For this review, take the finished solid that the model builds, in its own axes (mm). Face numbers are marked on the shaded views. A direction names the side the tool comes from. Round coordinates to 2 decimals unless told otherwise and drop trailing zeros. Write each loop counter-clockwise with the first axis right and the second up, starting at its lowest first coordinate (ties: lowest second). Pieces come first, ordered by that corner, then holes. Notation, with made-up numbers: M 9,81.5 L 24,81.5 A20 cw 24,114.5 Z; hole C 63.25,22 d5. An arc over 180 degrees is marked long. Answer in a Markdown table with one row per item.
Autodesk Fusion 360 part; units mm, degrees
sketch "Sketch1" plane through (0, 0, 0) normal (0, 0, 1) x (1, 0, 0)
  circle A0 centre (0, 0) radius 30
  line L0 (0, 0) -> (129, 0) construction
  circle A1 centre (129, 0) radius 20
  line L1 (-11.547, 20) -> (-23.094, 0)
  line L2 (-23.094, 0) -> (-11.547, -20)
  line L3 (-11.547, -20) -> (11.547, -20)
  line L4 (11.547, -20) -> (23.094, 0)
  line L5 (23.094, 0) -> (11.547, 20)
  line L6 (11.547, 20) -> (-11.547, 20)
  line L7 (0, 0) -> (0, 40) construction
  line L8 (129, 0) -> (129, 50) construction
  line L9 (129, 15) -> (114.7342, 4.6353)
  line L10 (114.7342, 4.6353) -> (120.1832, -12.1353)
  line L11 (120.1832, -12.1353) -> (137.8168, -12.1353)
  line L12 (137.8168, -12.1353) -> (143.2658, 4.6353)
  line L13 (143.2658, 4.6353) -> (129, 15)
  line L14 (28.2843, 10) -> (111.6795, 10)
  line L15 (28.2843, -10) -> (111.6795, -10)
  line L16 (30, 0) -> (109, 0) construction
  line L17 (69.5, 0) -> (69.5, 17.0528) construction
  line L18 (99.5, -5) -> (39.5, -5)
  line L19 (39.5, -5) -> (39.5, 5) construction
  line L20 (39.5, 5) -> (99.5, 5)
  line L21 (99.5, 5) -> (99.5, -5) construction
  line L22 (99.5, -5) -> (39.5, 5) construction
  line L23 (39.5, -5) -> (99.5, 5) construction
  arc A2 (39.5, 5) -> (39.5, -5) centre (39.5, 0) ccw
  arc A3 (99.5, -5) -> (99.5, 5) centre (99.5, 0) ccw
  point P0 (129, 0)
  point P1 (64.5, 0)
  point P2 (69.5, 0)
  dimension "d1" = 60
  dimension "d2" = 129
  dimension "d3" = 40
  dimension "d4" = 20
  dimension "d5" = 15
  dimension "d6" = 10
  dimension "d7" = 10
  dimension "d17" = 10
  dimension "d19" = 60
extrude "Extrude1" add sketch "Sketch1" along normal mid plane 20 contours A0 | A1 makes body 1 at (27.1662, -12.7278, 3.3333) makes body 2 at (148.9006, -1.9914, -3.3333)
extrude "Extrude2" add sketch "Sketch1" along normal mid plane 10 contours A0 A1 L14 L15 bodies 1 2
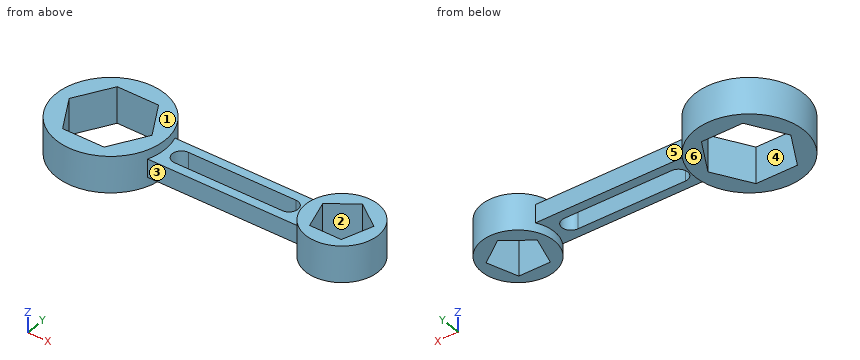
Q1. Take a section at D-D (x = 44). State the section outline as (y, z) points, then the cut area to 3 significant figures.
Found:
| item | result |
|---|---|
| outline | M -10,-5 L -5,-5 L -5,5 L -10,5 Z; M 5,-5 L 10,-5 L 10,5 L 5,5 Z |
| area | 100 mm² |
Q2. Mouldability with a two-part tool opening along X and no side actions: class the marked faces 1 and 2 as +X half, -X half, draft (parallel to the pull), parting line (faces both ways), or undercut.
Found:
| item | result |
|---|---|
| face 1 | draft |
| face 2 | undercut |
Q3. Take a section at B-B (x = 0). State the section outline as (y, z) points, then the cut area to 3 significant figures.
Found:
| item | result |
|---|---|
| outline | M -30,-10 L -20,-10 L -20,10 L -30,10 Z; M 20,-10 L 30,-10 L 30,10 L 20,10 Z |
| area | 400 mm² |
Q4. Machinability: for the marked faces 3, 4, 5 and 6, which of the approach directions +Z, -Z, +X, -X, +Y, -Y give a long, thin tool a straight path to every point of the face, cutting with its end or side? Answer none if there is none.
Found:
| item | result |
|---|---|
| face 3 | +Z, -Z, -Y |
| face 4 | +Z, -Z |
| face 5 | +Z, -Z, +Y |
| face 6 | -Z, +X, -X, +Y, -Y |
Q5. Take a section at A-A (z = -8.25). State the section outline as (x, y) points.
Found:
| item | result |
|---|---|
| outline | C 0,0 d60; C 129,0 d40; hole M -23.09,0 L -11.55,-20 L 11.55,-20 L 23.09,0 L 11.55,20 L -11.55,20 Z; hole M 114.73,4.64 L 120.18,-12.14 L 137.82,-12.14 L 143.27,4.64 L 129,15 Z |
Q6. Take a section at C-C (z = 3). State the section outline as (x, y) points, then the cut area to 3 significant figures.
Found:
| item | result |
|---|---|
| outline | M 28.28,-10 L 111.68,-10 A20 ccw long 111.68,10 L 28.28,10 A30 ccw long Z; hole M -23.09,0 L -11.55,-20 L 11.55,-20 L 23.09,0 L 11.55,20 L -11.55,20 Z; hole M 39.5,-5 L 99.5,-5 A5 ccw 99.5,5 L 39.5,5 A5 ccw Z; hole M 114.73,4.64 L 120.18,-12.14 L 137.82,-12.14 L 143.27,4.64 L 129,15 Z |
| area | 3,090 mm² |
Q7. For probe 1 along X at (y, z) = (-10, -8.5); probe 2 along X at (y, z) = (2, -4); probe 3 along Y at (x, z) = (82, 1), list the stretches that pass through material, from the lowest coordinate up.
Found:
| item | result |
|---|---|
| probe 1 | -28.28 to -17.32, 17.32 to 28.28, 111.68 to 119.49, 138.51 to 146.32 |
| probe 2 | -29.93 to -21.94, 21.94 to 34.92, 104.08 to 115.59, 142.41 to 148.9 |
| probe 3 | -10 to -5, 5 to 10 |
Q8. Insertion check: P1, Ø5, axis at y = 9.5, z = -3, coming from the +X side (3 decimals); P2, Ø6, axis at x = 2.5, z = -1.5, coming from the +Y side; P3, Ø5, axis at x = 106.5, y = -6, coming from the +Z side. Each pin has a flat end and moves straight along its axis. Give the tip position at first contact, or say it passes through.
Found:
| item | result |
|---|---|
| P1 | x = 147.735 |
| P2 | y = 30 |
| P3 | z = 5 |
